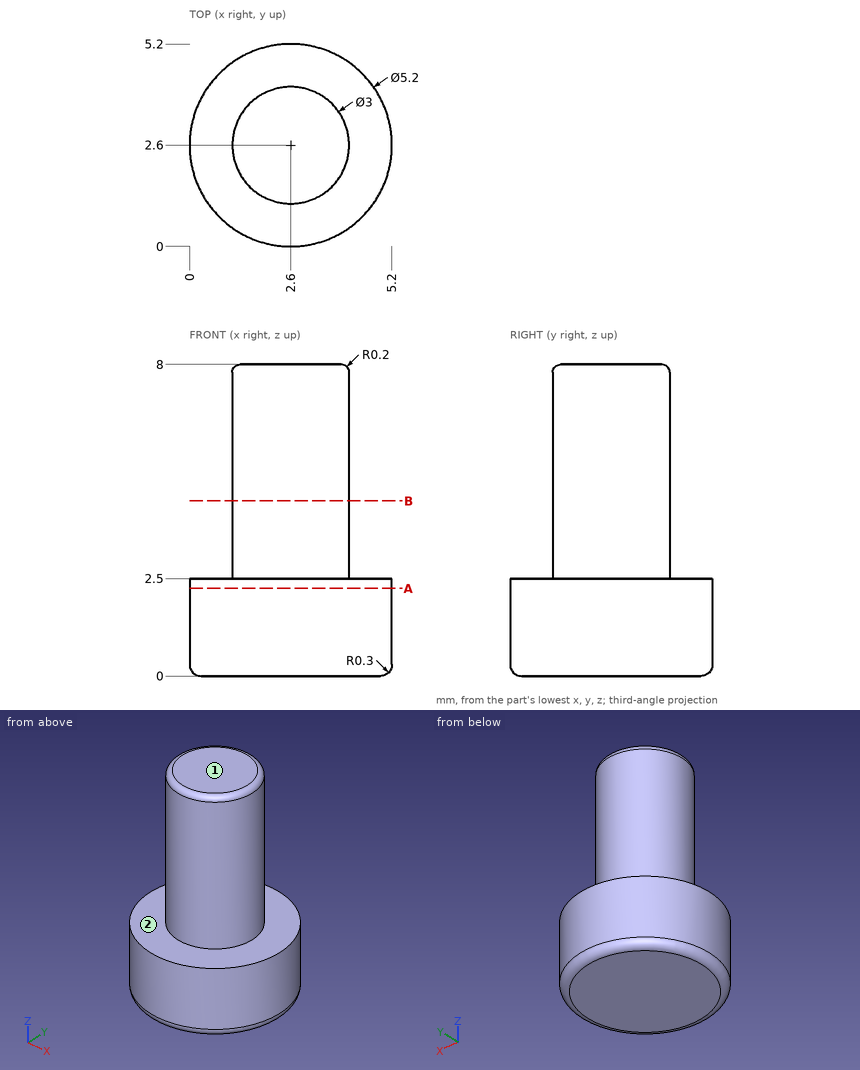
Study the drawing (mm; zero at the part's minimum x, y, z) and answer. A direction names the side the tool comes from. Give positions to 0.01 mm unless a question says otherwise; leave off trailing zeros. Write each loop counter-clockwise with the first axis right and the second up, starting at its lowest first coordinate (ties: lowest second). Pieces come first, ordered by that corner, then holes. Notation, with made-up numbers: (-21.75, 49.5) -> (13.25, 49.5) arc R24 ccw to (13.25, 79.5) -> close; hole circle Ø2 at (1, 33). An arc over 180 degrees is marked (long way). Answer as a JSON object with one key per item and string values. Group by question number.
1) Consider L1, parallel to Y at x = 2.5, z = 1.25; L2, parallel to Z at x = 0.3, y = 2.5; L3, parallel to X at y = 1.9, z = 4. Determine where each line is inside the solid, lowest interval first. Write a range as from..to.
2) Each of these flat-tipped pins is pushed along its axis until it touches: P1, Ø2, axis at x = 4, z = 1.5, coming from the +Y side; P2, Ø2, axis at y = 2.5, z = 4.5, coming from the +X side; P3, Ø1.5, axis at x = 1.5, z = 5.5, coming from the -Y side. Where does it stop, or does it pass through?
3) Find section A-A (z = 2.25). Write down the section's boundary in (x, y).
4) A tool of negligible diameter and unlimited length cuts with its end or side. For the marked faces 1 and 2, from which of +Z, -Z, +X, -X, +Y, -Y can it reach the whole face along a straight path? Write none if from no direction.
5) Find section B-B (z = 4.5). Write down the section's boundary in (x, y), and give its area (3 significant figures).
Values follow:
{
 "1": {"L1": "y = 0..5.2", "L2": "z = 0..2.5", "L3": "x = 1.27..3.93"},
 "2": {"P1": "stops at y = 5.17", "P2": "stops at x = 4.1", "P3": "stops at y = 1.14"},
 "3": {"outline": "circle Ø5.2 at (2.6, 2.6)"},
 "4": {"face 1": "+Z, +X, -X, +Y, -Y", "face 2": "+Z"},
 "5": {"outline": "circle Ø3 at (2.6, 2.6)", "area": "7.07 mm2"}
}
